```python
from build123d import *

# Parameters (mm, degrees)
F3_W     = 92.075
F3_H     = 193.675
F4_DEPTH = 355.6
F0_D     = 12.7
F0_DEPTH = 101.601
F2_D     = 12.7
F2_DEPTH = 101.601
F6_D     = 6.35
F6_DEPTH = 101.601


with BuildPart() as f4:
    # F3 (on Front) → F4 (new body)
    with BuildSketch(Plane.XZ):
        with BuildLine():
            ThreePointArc((-50.8, -95.25), (-48.9401280605, -99.7401280605), (-44.45, -101.6))
            Line((-44.45, -101.6), (44.45, -101.6))
            ThreePointArc((44.45, -101.6), (48.9401280605, -99.7401280605), (50.8, -95.25))
            Line((50.8, -95.25), (50.8, 95.25))
            ThreePointArc((50.8, 95.25), (48.9401280605, 99.7401280605), (44.45, 101.6))
            Line((44.45, 101.6), (-44.45, 101.6))
            ThreePointArc((-44.45, 101.6), (-48.9401280605, 99.7401280605), (-50.8, 95.25))
            Line((-50.8, 95.25), (-50.8, -95.25))
        make_face()
        Rectangle(F3_W, F3_H, mode=Mode.SUBTRACT)
    extrude(amount=-F4_DEPTH)

    # F0 (through all, one way)
    with BuildSketch(Plane.XY):
        with Locations((0, 228.6), (0, 152.4), (0, 76.2)):
            Circle(F0_D / 2)
    extrude(amount=-F0_DEPTH, mode=Mode.SUBTRACT)

    # F2 (through all, one way)
    with BuildSketch(Plane(origin=(0, 0, 0), x_dir=(1, 0, 0), z_dir=(0, 0, -1))):
        with Locations((-25.4, -165.1)):
            Circle(F2_D / 2)
    extrude(amount=-F2_DEPTH, mode=Mode.SUBTRACT)

    # F6 (through all, one way)
    with BuildSketch(Plane(origin=(0, 0, 0), x_dir=(1, 0, 0), z_dir=(0, 0, -1))):
        with Locations((31.75, -12.7), (-31.75, -12.7), (-31.75, -50.8), (31.75, -50.8), (19.05, -139.7), (-19.05, -139.7), (19.05, -120.65), (-19.05, -120.65)):
            Circle(F6_D / 2)
    extrude(amount=-F6_DEPTH, mode=Mode.SUBTRACT)


solid = f4.part
```
CAD build for the part. Positions are in the model's coordinates, mm. A direction names the side the tool comes from. Give positions to 0.01 mm unless a question says otherwise; leave off trailing zeros. Loops run counter-clockwise (first coordinate to the right, second up) from the corner with the lowest first, then second, coordinate; pieces in that order, holes last. Notation, with made-up numbers: (-29.5, 33) -> (-21.5, 33) arc R31 cw to (-21.5, 72) -> close; hole circle Ø2 at (-24.5, -21). An arc over 180 degrees is marked (long way). Use a Markdown table: item, result.
1. Which spindle directions (+Z, -Z, +X, -X, +Y, -Y) get a long thin tool onto all of the face, cutting with end or side? Do faces 1 (the cylindrical face through (-48.99, 175.31, -99.69)), 2 (the cylindrical face through (31.06, 15.8, 99.19)), 3 (the flat face through (-1, 175, -96.838)), 4 (the cylindrical face through (48.99, 175.31, 99.69)), 5 (the cylindrical face through (-1.38, 222.4, -99.19)). Say none if no direction does.
Check result:
| item | result |
|---|---|
| face 1 | -Z, -X, +Y, -Y |
| face 2 | +Z |
| face 3 | +Y, -Y |
| face 4 | +Z, +X, +Y, -Y |
| face 5 | -Z |
2. Flat gauge pins, fed straight in: pin 1 (4 mm diameter, centred on x = 19.05, y = 120.65, fed in from +Z); pin 2 (7.5 mm diameter, centred on x = 0, y = 152.4, fed in from -Z). Where does each tip first touch, or does it go through?
Check result:
| item | result |
|---|---|
| pin 1 | stops at z = -96.84 |
| pin 2 | stops at z = 96.84 |
3. Wall check: L1, parallel to Y at x = 31.75, z = 100.65 (3 decimals); L2, parallel to Y at x = -25, z = 100; L3, parallel to Z at x = -31, y = 37.5. Give the ranges that are in metal, low to high. Write a range as [from, to].
Check result:
| item | result |
|---|---|
| L1 | y = [0, 9.525], [15.875, 47.625], [53.975, 355.6] |
| L2 | y = [0, 158.76], [171.44, 355.6] |
| L3 | z = [-101.6, -96.84], [96.84, 101.6] |
4. Slice it at B-B (y = 186). List the corners of the cut face in (x, z), plus the area to 3 significant figures.
Check result:
| item | result |
|---|---|
| outline | (-50.8, -95.25) arc R6.35 ccw to (-44.45, -101.6) -> (44.45, -101.6) arc R6.35 ccw to (50.8, -95.25) -> (50.8, 95.25) arc R6.35 ccw to (44.45, 101.6) -> (-44.45, 101.6) arc R6.35 ccw to (-50.8, 95.25) -> close; hole (-46.04, -96.84) -> (46.04, -96.84) -> (46.04, 96.84) -> (-46.04, 96.84) -> close |
| area | 2,780 mm^2 |
5. Slice it at C-C (z = -25). List the corners of the cut face in (x, y).
Check result:
| item | result |
|---|---|
| outline | (-50.8, 0) -> (-46.04, 0) -> (-46.04, 355.6) -> (-50.8, 355.6) -> close; (46.04, 0) -> (50.8, 0) -> (50.8, 355.6) -> (46.04, 355.6) -> close |
6. Slice it at A-A (x = 0). List the corners of the cut face in (y, z), plus the area to 3 significant figures.
Check result:
| item | result |
|---|---|
| outline | (0, -101.6) -> (69.85, -101.6) -> (69.85, -96.84) -> (0, -96.84) -> close; (0, 96.84) -> (355.6, 96.84) -> (355.6, 101.6) -> (0, 101.6) -> close; (82.55, -101.6) -> (146.05, -101.6) -> (146.05, -96.84) -> (82.55, -96.84) -> close; (158.75, -101.6) -> (222.25, -101.6) -> (222.25, -96.84) -> (158.75, -96.84) -> close; (234.95, -101.6) -> (355.6, -101.6) -> (355.6, -96.84) -> (234.95, -96.84) -> close |
| area | 3,210 mm^2 |
7. Mould opens along Z. For faces 6 (the flat face through (-1, 175, 96.838)), 7 (the flat face through (1, 175, 101.6)), 8 (the cylindrical face through (48.89, 175.31, -99.79)) say: pulls with the +Z half, pulls with the -Z half, needs draft (parallel to the pull), parting line crosses it, or undercut.
Check result:
| item | result |
|---|---|
| face 6 | undercut |
| face 7 | pulls with the +Z half |
| face 8 | pulls with the -Z half |
